Check sheet for the modelled part. Datum: model origin and axes. Units: mm. Give positions to 0.01 mm unless a question says otherwise; leave off trailing zeros. Loops run counter-clockwise (first coordinate to the right, second up) from the corner with the lowest first, then second, coordinate; pieces in that order, holes last.
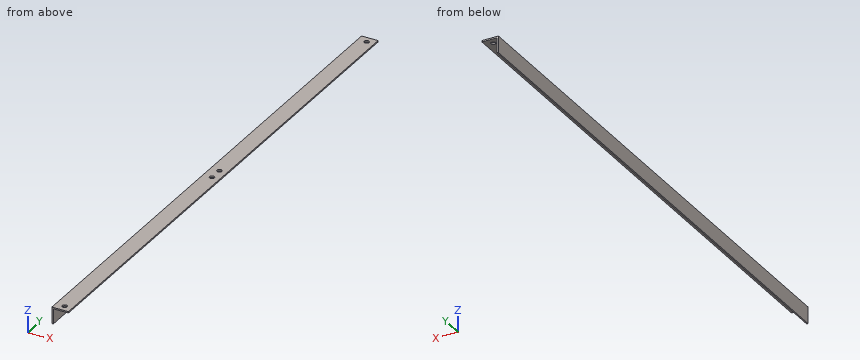
```python
from build123d import *

# Parameters (mm, degrees)
BOSS_EXTRUDE1_DEPTH = 635
SKETCH19_R          = 5.588
CUT_EXTRUDE2_DEPTH  = 638.099965174


with BuildPart() as part:
    # Sketch18 → Boss-Extrude1 (new, symmetric)
    with BuildSketch(Plane(origin=(0, 0, 0), x_dir=(1, 0, 0), z_dir=(0, 1, 0))):
        Polygon((3.175, 38.1), (3.175, 3.175), (38.1, 3.175), (38.1, 0), (0, 0), (0, 38.1), align=None)
    extrude(amount=BOSS_EXTRUDE1_DEPTH, both=True)

    # Sketch19 → Cut-Extrude2 (cut, through all)
    with BuildSketch(Plane(origin=(0, 0, -3.175), x_dir=(-1, 0, 0), z_dir=(0, 0, -1))):
        with Locations((-20.6375, 619.125)):
            Circle(SKETCH19_R)
        with Locations((-20.6375, 15.24)):
            Circle(SKETCH19_R)
    cut_extrude2 = extrude(amount=-CUT_EXTRUDE2_DEPTH, mode=Mode.SUBTRACT)

    # Mirror2: Cut-Extrude2 across plane
    add(cut_extrude2.mirror(Plane.ZX), mode=Mode.SUBTRACT)


solid = part.part
```
(1) Section check A-A on y = 362. Record the boundary of the cut face in (x, z) (3 decimals), plus the area to 3 significant figures.
(2) Gauge pin test, flat ends, axial feed: pin 1 Ø3 at (x, z) = (32.5, -6) entering from +Y; pin 2 Ø10 at (x, y) = (18.5, -130.5) entering from -Z (3 decimals); pin 3 Ø12 at (y, z) = (-48, -13.5) entering from +X (3 decimals). Record the tip position at first contact, or that the pin passes through.
(3) Section check B-B on z = -14. Record the boundary of the cut face in (x, y) (3 decimals).
(4) Material ranges on line 1 (X direction, y = -15.24, z = -2.3); line 2 (Z direction, x = 6.5, y = -580) (3 decimals); line 3 (X direction, y = 416, z = -12.5) (3 decimals), recorded low to high.
Computed values:
1. outline: (0, -38.1) - (3.175, -38.1) - (3.175, -3.175) - (38.1, -3.175) - (38.1, 0) - (0, 0) - close
1. area: 232 mm2
2. pin 1: passes through
2. pin 2: stops at z = -3.175
2. pin 3: stops at x = 3.175
3. outline: (0, -635) - (3.175, -635) - (3.175, 635) - (0, 635) - close
4. line 1: x = 0 to 15.05, 26.23 to 38.1
4. line 2: z = -3.175 to 0
4. line 3: x = 0 to 3.175
